The model under review builds one solid part; all positions refer to its coordinate system, in mm. A direction names the side the tool comes from. Coordinates: 2 decimals unless noted, no trailing zeros. Order: outer loops, then holes, each group sorted by start corner. A loop starts at its lowest first (then second) coordinate and runs counter-clockwise, first axis right, second up. Notation, with made-up numbers: (9, -8) -> (30, -8) arc R15 cw to (30, 21) -> close; hole circle Ø11 at (56, 17.25). An arc over 180 degrees is marked (long way). Use one line per item in the form item = value. Start each with the question number.
(1) Take a section at C-C (y = 0). State the section outline as (x, z) points, then the cut area to 3 significant figures.
(2) Wall thickness on line 1 along Y through (x, z) = (251.5, 295); line 2 along Z through (x, y) = (418, 42.5); line 3 along Y through (x, z) = (-119.5, -3): over which ranges is each line inside the solid? List them lowest first.
(3) Take a section at B-B (x = 0). State the section outline as (y, z) points.
(4) Take a section at A-A (z = 582.5). State the section outline as (x, y) points.
(5) Insertion check: pin 1 Ø10 at (x, y) = (-185, 312.5) entering from +Z; pin 2 Ø25 at (y, z) = (-251.5, 419) entering from +X; pin 3 Ø1.5 at (x, y) = (196.5, 80) entering from -Z; pin 4 Ø1.5 at (x, z) = (276.5, 242) entering from -Y. Each pin has a flat end and moves straight along its axis. Give the tip position at first contact, or say it passes through.
(6) Take a section at D-D (x = 241.5). State the section outline as (y, z) points, then the cut area to 3 significant figures.
(7) Mouldability with a two-part tool opening along X and no side actions: class faces 1 (the flat face through (-250, -250, 700)), 2 (the flat face through (275, -250, 370)), 3 (the flat face through (-225, -250, 370)), 4 (the flat face through (-2, 275, 99)) as +X half, -X half, draft (parallel to the pull), parting line (faces both ways), or undercut.
(8) For faces 5 (the flat face through (-225, 250, 370)), 6 (the flat face through (-2, 475, 99)), 7 (the flat face through (-250, -225, 370)), list the 3-axis set-ups (+Z, -Z, +X, -X, +Y, -Y) from which the entire face can be reached by the end or side of a thin tool; tool diameter is ignored.
```python
from build123d import *

# Parameters (mm, degrees)
SKETCH_1_R      = 500
EXTRUDE_1_DEPTH = 50
SKETCH_2_W      = 50
SKETCH_2_H      = 50
EXTRUDE_2_DEPTH = 700
SKETCH_3_W      = 50
SKETCH_3_H      = 50
EXTRUDE_3_DEPTH = 700
SKETCH_4_W      = 50
SKETCH_4_H      = 50
EXTRUDE_4_DEPTH = 700
SKETCH_5_W      = 50
SKETCH_5_H      = 50
EXTRUDE_5_DEPTH = 700
SKETCH_6_W      = 300
SKETCH_6_H      = 300
EXTRUDE_6_DEPTH = 200


with BuildPart() as part:
    # 草图1 → 凸台-拉伸1 (new body)
    with BuildSketch(Plane.XY):
        Circle(SKETCH_1_R)
    extrude(amount=EXTRUDE_1_DEPTH)

    # 草图2 → 凸台-拉伸2 (add)
    with BuildSketch(Plane.XY):
        with Locations((250, 250)):
            Rectangle(SKETCH_2_W, SKETCH_2_H)
    extrude(amount=EXTRUDE_2_DEPTH)

    # 草图3 → 凸台-拉伸3 (add)
    with BuildSketch(Plane.XY):
        with Locations((-250, 250)):
            Rectangle(SKETCH_3_W, SKETCH_3_H)
    extrude(amount=EXTRUDE_3_DEPTH)

    # 草图4 → 凸台-拉伸4 (add)
    with BuildSketch(Plane.XY):
        with Locations((250, -250)):
            Rectangle(SKETCH_4_W, SKETCH_4_H)
    extrude(amount=EXTRUDE_4_DEPTH)

    # 草图5 → 凸台-拉伸5 (add)
    with BuildSketch(Plane.XY):
        with Locations((-250, -250)):
            Rectangle(SKETCH_5_W, SKETCH_5_H)
    extrude(amount=EXTRUDE_5_DEPTH)

    # 草图6 → 凸台-拉伸6 (add)
    with BuildSketch(Plane(origin=(0, 275, 0), x_dir=(1, 0, 0), z_dir=(0, 1, 0))):
        Rectangle(SKETCH_6_W, SKETCH_6_H)
    extrude(amount=EXTRUDE_6_DEPTH)


solid = part.part
```
Findings:
q1.outline = (-500, 0) -> (500, 0) -> (500, 50) -> (-500, 50) -> close
q1.area = 50,000 mm²
q2.line_1 = -275 to -225, 225 to 275
q2.line_2 = 0 to 50
q2.line_3 = 275 to 475
q3.outline = (-500, 0) -> (275, 0) -> (275, -150) -> (475, -150) -> (475, 0) -> (500, 0) -> (500, 50) -> (475, 50) -> (475, 150) -> (275, 150) -> (275, 50) -> (-500, 50) -> close
q4.outline = (-275, -275) -> (-225, -275) -> (-225, -225) -> (-275, -225) -> close; (-275, 225) -> (-225, 225) -> (-225, 275) -> (-275, 275) -> close; (225, -275) -> (275, -275) -> (275, -225) -> (225, -225) -> close; (225, 225) -> (275, 225) -> (275, 275) -> (225, 275) -> close
q5.pin_1 = 50
q5.pin_2 = 275
q5.pin_3 = 0
q5.pin_4 = through
q6.outline = (-437.81, 0) -> (437.81, 0) -> (437.81, 50) -> (275, 50) -> (275, 700) -> (225, 700) -> (225, 50) -> (-225, 50) -> (-225, 700) -> (-275, 700) -> (-275, 50) -> (-437.81, 50) -> close
q6.area = 109,000 mm²
q7.face_1 = draft
q7.face_2 = +X half
q7.face_3 = undercut
q7.face_4 = undercut
q8.face_5 = +Z, +Y, -Y
q8.face_6 = +Z, +X, -X, +Y
q8.face_7 = +Z, +X, -X
